Autodesk Inventor part; units mm, degrees
ref_plane "YZ Plane" through (0, 0, 0) normal (1, 0, 0) x (0, 1, 0)
ref_plane "XZ Plane" through (0, 0, 0) normal (0, 1, 0) x (-1, 0, 0)
ref_plane "XY Plane" through (0, 0, 0) normal (0, 0, 1) x (1, 0, 0)
sketch "Sketch1" plane through (0, 0, 0) normal (0, 0, 1) x (1, 0, 0)
  line L0 (-300, -275) -> (300, -275)
  line L1 (300, -275) -> (300, 275)
  line L2 (300, 275) -> (-300, 275)
  line L3 (-300, 275) -> (-300, -275)
  line L4 (-300, -275) -> (300, 275) construction
  line L5 (300, -275) -> (-300, 275) construction
  line L6 (-150, -80) -> (150, -80)
  line L7 (150, -80) -> (150, 120)
  line L8 (150, 120) -> (-150, 120)
  line L9 (-150, 120) -> (-150, -80)
  line L10 (-150, -80) -> (150, 120) construction
  line L11 (150, -80) -> (-150, 120) construction
  line L12 (0, 20) -> (0, 0) construction
  dimension "d0" = 600
  dimension "d1" = 550
  dimension "d4" = 300
  dimension "d5" = 200
  dimension "d6" = 20
extrude "Extrusion1" add sketch "Sketch1" along normal blind 6
properties part number "drzwiczki-przod"
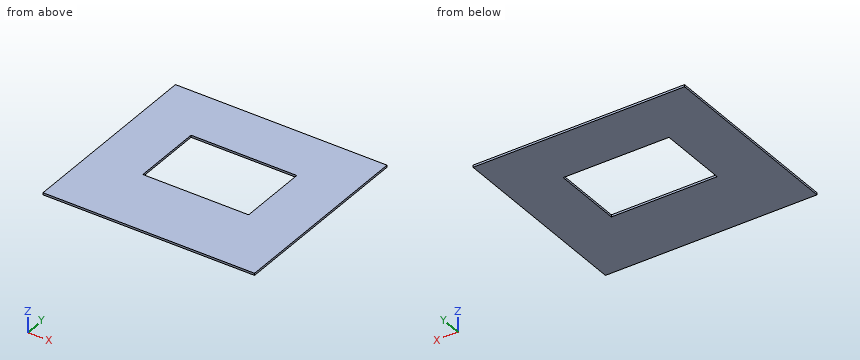
CAD build for the part. Positions are in the model's coordinates, mm. Round coordinates to 2 decimals unless told otherwise and drop trailing zeros. Write each loop counter-clockwise with the first axis right and the second up, starting at its lowest first coordinate (ties: lowest second). Pieces come first, ordered by that corner, then holes. Notation, with made-up numbers: (81, 84.25) -> (114, 84.25) arc R18 ccw to (114, 117.25) -> close; hole circle Ø1 at (31.25, 7.5). An arc over 180 degrees is marked (long way). Answer in a Markdown table with one row per item. Add a question column.
Item 1: Saw through at C-C, the plane z = 2.8. Write the cut outline in (x, y).
Item 2: Saw through at B-B, the plane y = -67.5. Write the cut outline in (x, z).
Item 3: Saw through at A-A, the plane x = -133. Write the cut outline in (y, z).
Item 4: Drill centre lines: line 1 (X direction, y = 65, z = 3.1); line 2 (Y direction, x = -60, z = 2.1). Where is each one in solid material? Low to high. Write a range as from..to.
Item 5: Drop a flat-ended pin along its axis: pin 1 Ø3 at (x, y) = (-238.5, -16) entering from -Z. Give the stop position or say it passes through.
Findings below:
| question | item | result |
|---|---|---|
| 1 | outline | (-300, -275) -> (300, -275) -> (300, 275) -> (-300, 275) -> close; hole (-150, -80) -> (150, -80) -> (150, 120) -> (-150, 120) -> close |
| 2 | outline | (-300, 0) -> (-150, 0) -> (-150, 6) -> (-300, 6) -> close; (150, 0) -> (300, 0) -> (300, 6) -> (150, 6) -> close |
| 3 | outline | (-275, 0) -> (-80, 0) -> (-80, 6) -> (-275, 6) -> close; (120, 0) -> (275, 0) -> (275, 6) -> (120, 6) -> close |
| 4 | line 1 | x = -300..-150, 150..300 |
| 4 | line 2 | y = -275..-80, 120..275 |
| 5 | pin 1 | stops at z = 0 |
